Check sheet for the modelled part. Datum: model origin and axes. Units: mm. A direction names the side the tool comes from. Coordinates: 2 decimals unless noted, no trailing zeros. Order: outer loops, then holes, each group sorted by start corner. A loop starts at its lowest first (then second) coordinate and runs counter-clockwise, first axis right, second up.
from build123d import *

# Parameters (mm, degrees)
F1_DEPTH = 88.9
F2_DEPTH = 19.05
F3_R     = 39.6875
F4_DEPTH = 7.62


with BuildPart() as f1:
    # F0 (on Top) → F1 (new body)
    with BuildSketch(Plane.XY):
        Polygon((0, -76.2), (0, -1016), (406.4, -1016), (1016, -406.4), (1016, 0), (76.2, 0), align=None)
        Polygon((398.509232, -996.95), (19.05, -996.95), (19.05, -84.090768), (84.090768, -19.05), (996.95, -19.05), (996.95, -398.509232), align=None, mode=Mode.SUBTRACT)
    extrude(amount=-F1_DEPTH)

    # F0 (on Top) → F2 (join)
    with BuildSketch(Plane.XY):
        Polygon((19.05, -84.090768), (19.05, -996.95), (398.509232, -996.95), (996.95, -398.509232), (996.95, -19.05), (84.090768, -19.05), align=None)
    extrude(amount=-F2_DEPTH)

    # F3 (on face) → F4 (join)
    with BuildSketch(Plane(origin=(0, 0, -19.05), x_dir=(1, 0, 0), z_dir=(0, 0, -1))):
        with Locations((76.2, 939.8)):
            Circle(F3_R)
        with Locations((91.981537, 91.981537)):
            Circle(F3_R)
        with Locations((374.836927, 939.8)):
            Circle(F3_R)
        with Locations((939.8, 374.836927)):
            Circle(F3_R)
        with Locations((939.8, 76.2)):
            Circle(F3_R)
    extrude(amount=F4_DEPTH)


solid = f1.part
(1) Release check for a two-part mould opening along Y. For faces 3 (the flat face through (388, -388, 0)), 4 (the flat face through (553, 0, -44)), 5 (the flat face through (996.95, -206, -53)), 6 (the cylindrical face through (369.67, -979.15, -22.81)) record: +Y half, -Y half, draft (parallel to the pull), parting line (faces both ways), or undercut.
Filled in:
face 3: draft
face 4: +Y half
face 5: undercut
face 6: undercut
(2) Thickness scan on probe 1 along Y at (x, z) = (393, -73); probe 2 along X at (y, z) = (-259, -31.5); probe 3 along Z at (x, y) = (927.5, -308). Record the ranges inside material, lowest first.
Filled in:
probe 1: y = -1016 to -996.95, -19.05 to 0
probe 2: x = 0 to 19.05, 996.95 to 1016
probe 3: z = -19.05 to 0
(3) Cross-section at D-D (x = 939.8). Enter the section's corners in (y, z), and give its area (3 significant figures).
Filled in:
outline: (-482.6, -88.9) - (-455.66, -88.9) - (-455.66, -19.05) - (-414.52, -19.05) - (-414.52, -26.67) - (-335.15, -26.67) - (-335.15, -19.05) - (-115.89, -19.05) - (-115.89, -26.67) - (-36.51, -26.67) - (-36.51, -19.05) - (-19.05, -19.05) - (-19.05, -88.9) - (0, -88.9) - (0, 0) - (-482.6, 0) - close
area: 13,600 mm2
(4) Cross-section at C-C (y = -706). Enter the section's corners in (x, z).
Filled in:
outline: (0, -88.9) - (19.05, -88.9) - (19.05, -19.05) - (689.46, -19.05) - (689.46, -88.9) - (716.4, -88.9) - (716.4, 0) - (0, 0) - close
(5) Go/stop test with flat-tipped pins: P1, Ø21, axis at x = 539.5, z = -59, coming from the -Y side; P2, Ø24, axis at x = 369.5, y = -948, coming from the -Z side; P3, Ø5, axis at y = -808, z = -78, coming from the +X side. Record where each tip stops, or that it passes through.
Filled in:
P1: stops at y = -893.4
P2: stops at z = -26.67
P3: stops at x = 616.9
(6) Cross-section at B-B (x = 244). Enter the section's corners in (y, z).
Filled in:
outline: (-1016, -88.9) - (-996.95, -88.9) - (-996.95, -19.05) - (-19.05, -19.05) - (-19.05, -88.9) - (0, -88.9) - (0, 0) - (-1016, 0) - close
(7) Tool access check on faces 1 (the flat face through (38.6, -37.6, -43.8)), 2 (the cylindrical face through (961.14, -408.3, -22.81)). Record the directions out of +Z, -Z, +X, -X, +Y, -Y that give a thin tool (end or side, any length) a straight path to the whole face; none if there is none.
Filled in:
face 1: +Z, -Z, -X, +Y
face 2: -Z
(8) Cross-section at A-A (z = -63.5). Enter the section's corners in (x, y).
Filled in:
outline: (0, -1016) - (406.4, -1016) - (1016, -406.4) - (1016, 0) - (76.2, 0) - (0, -76.2) - close; hole (19.05, -996.95) - (398.51, -996.95) - (996.95, -398.51) - (996.95, -19.05) - (84.09, -19.05) - (19.05, -84.09) - close
